Build history of the part. All positions in model axes, mm. A direction names the side the tool comes from. Coordinates: 2 decimals unless noted, no trailing zeros. Loops run counter-clockwise (first coordinate to the right, second up) from the corner with the lowest first, then second, coordinate; pieces in that order, holes last.
(1) Slice it at C-C (y = 17). Give the cut face in (x, z), and give its area (3 significant figures).
(2) Flat gauge pins, fed straight in: P1, Ø1, axis at x = 5, z = 4, coming from the -Y side; P2, Ø3, axis at x = -40.5, z = 6.5, coming from the -Y side; P3, Ø3, axis at x = -32, z = 7.5, coming from the +Y side. Where does each tip first touch, or does it go through?
(3) Slice it at B-B (z = 5). Give the number of separate pieces and of enclosed holes in the cut face, and give its area (3 significant figures).
(4) Slice it at A-A (x = 0). Give the cut face in (y, z).
(5) Slice it at D-D (x = 12.5). Give the cut face in (y, z).
(6) Two-plate mould, pull along Y, no slides. Class faces 5 (the face through (7.17, -39.42, 4.93)), 6 (the face through (30.656, -26.098, 4.93)), 7 (the face through (20, -1, 0)), 8 (the face through (12.03, 37.84, 4.93)): pulls with the +Y half, pulls with the -Y half, needs draft (parallel to the pull), parting line crosses it, or undercut.
(7) Tool access for faces 1 (the face through (22.336, -39.066, 4.93)), 2 (the face through (26.67, 29.19, 4.93)), 3 (the face through (-39, -8.5, 5)), 4 (the face through (-15, 19.8, 5.1)): list every direction of +Z, -Z, +X, -X, +Y, -Y with a clear straight run to the whole face (end or side of a thin tool).
(8) Wall check: L1, parallel to Y at x = -3.5, z = 6; L2, parallel to X at y = -23.5, z = 5.75; L3, parallel to X at y = 1, z = 7.5. Give the ranges that are in metal, low to high.
from build123d import *

# Parameters (mm, degrees)
SALIENTE_EXTRUIR3_DEPTH = 10
CROQUIS2_R              = 16
CROQUIS2_R_2            = 4
CROQUIS2_R_3            = 3.3
CORTAR_EXTRUIR1_DEPTH   = 65.926288457


with BuildPart() as part:
    # Croquis1 → Saliente-Extruir3 (new body)
    with BuildSketch(Plane.XY):
        with BuildLine():
            Line((-45, -8.5), (-32.403703492, -8.5))
            ThreePointArc((-32.403703492, -8.5), (-33.5, 0), (-32.403703492, 8.5))
            Line((-32.403703492, 8.5), (-45, 8.5))
            Line((-45, 8.5), (-45, -8.5))
        make_face()
        with BuildLine():
            ThreePointArc((-32.403703492, 8.5), (-33.5, 0), (-32.403703492, -8.5))
            Line((-32.403703492, -8.5), (-30, -8.5))
            Line((-30, -8.5), (-30, 8.5))
            Line((-30, 8.5), (-32.403703492, 8.5))
        make_face()
        with BuildLine():
            Line((3.308657049, -32.730762114), (26.691342951, -19.230762114))
            Line((26.691342951, -19.230762114), (27.021052668, -19.801836095))
            ThreePointArc((27.021052668, -19.801836095), (31.839089688, -10.417406962), (33.5, 0))
            ThreePointArc((33.5, 0), (30.916118508, 12.901302895), (23.563067678, 23.812430401))
            Line((23.563067678, 23.812430401), (22.361215932, 21.730762114))
            Line((22.361215932, 21.730762114), (7.638784068, 30.230762114))
            Line((7.638784068, 30.230762114), (8.840635814, 32.312430401))
            ThreePointArc((8.840635814, 32.312430401), (-16.75, 29.011851027), (-32.403703492, 8.5))
            Line((-32.403703492, 8.5), (-30, 8.5))
            Line((-30, 8.5), (-30, -8.5))
            Line((-30, -8.5), (-32.403703492, -8.5))
            ThreePointArc((-32.403703492, -8.5), (-18.9906271, -27.597211496), (3.638366766, -33.301836095))
            Line((3.638366766, -33.301836095), (3.308657049, -32.730762114))
        make_face()
        with BuildLine():
            Line((22.361215932, 21.730762114), (23.563067678, 23.812430401))
            ThreePointArc((23.563067678, 23.812430401), (16.75, 29.011851027), (8.840635814, 32.312430401))
            Line((8.840635814, 32.312430401), (7.638784068, 30.230762114))
            Line((7.638784068, 30.230762114), (22.361215932, 21.730762114))
        make_face()
        with BuildLine():
            ThreePointArc((8.840635814, 32.312430401), (16.75, 29.011851027), (23.563067678, 23.812430401))
            Line((23.563067678, 23.812430401), (29.861215932, 34.72114317))
            Line((29.861215932, 34.72114317), (15.138784068, 43.22114317))
            Line((15.138784068, 43.22114317), (8.840635814, 32.312430401))
        make_face()
        with BuildLine():
            Line((27.021052668, -19.801836095), (26.691342951, -19.230762114))
            Line((26.691342951, -19.230762114), (3.308657049, -32.730762114))
            Line((3.308657049, -32.730762114), (3.638366766, -33.301836095))
            ThreePointArc((3.638366766, -33.301836095), (16.75, -29.011851027), (27.021052668, -19.801836095))
        make_face()
        with BuildLine():
            Line((34.191342951, -32.22114317), (27.021052668, -19.801836095))
            ThreePointArc((27.021052668, -19.801836095), (16.75, -29.011851027), (3.638366766, -33.301836095))
            Line((3.638366766, -33.301836095), (10.808657049, -45.72114317))
            Line((10.808657049, -45.72114317), (34.191342951, -32.22114317))
        make_face()
    extrude(amount=SALIENTE_EXTRUIR3_DEPTH)

    # Croquis2 → Cortar-Extruir1 (cut, through all)
    with BuildSketch(Plane.XY.offset(10)):
        Circle(CROQUIS2_R)
        with Locations((12.5, -21.650635095)):
            Circle(CROQUIS2_R_2)
        with Locations((24.148145657, -6.470476128)):
            Circle(CROQUIS2_R_3)
        with Locations((-6.470476128, -24.148145657)):
            Circle(CROQUIS2_R_3)
        with Locations((6.470476128, 24.148145657)):
            Circle(CROQUIS2_R_3)
        with Locations((-24.148145657, 6.470476128)):
            Circle(CROQUIS2_R_3)
        with Locations((24.947836968, -29.091113341)):
            Circle(CROQUIS2_R_3)
        with Locations((12.719724694, -36.151017254)):
            Circle(CROQUIS2_R_3)
        Polygon((-19.486906027, 27.568394577), (-10.486906027, 11.979937309), (-5.213138932, 15.024748161), (-14.213138932, 30.613205429), align=None)
        with Locations((-38.701851746, 0)):
            Circle(CROQUIS2_R_3)
        with Locations((19.350925873, 33.516786786)):
            Circle(CROQUIS2_R_3)
    extrude(amount=-CORTAR_EXTRUIR1_DEPTH, mode=Mode.SUBTRACT)


solid = part.part
Response values:
1. outline: (-28.87, 0) - (-13.39, 0) - (-13.39, 10) - (-28.87, 10) - close; (-6.35, 0) - (28.87, 0) - (28.87, 10) - (-6.35, 10) - close
1. area: 507 mm2
2. P1: stops at y = -36.53
2. P2: stops at y = -8.5
2. P3: stops at y = 13.86
3. separate pieces: 1
3. enclosed holes: 9
3. area: 3,030 mm2
4. outline: (-33.5, 0) - (-16, 0) - (-16, 10) - (-33.5, 10) - close; (16, 0) - (33.5, 0) - (33.5, 10) - (16, 10) - close
5. outline: (-44.74, 0) - (-39.44, 0) - (-39.44, 10) - (-44.74, 10) - close; (-32.86, 0) - (-25.65, 0) - (-25.65, 10) - (-32.86, 10) - close; (-17.65, 0) - (-9.99, 0) - (-9.99, 10) - (-17.65, 10) - close; (9.99, 0) - (38.65, 0) - (38.65, 10) - (9.99, 10) - close
6. face 5: pulls with the -Y half
6. face 6: undercut
6. face 7: needs draft
6. face 8: pulls with the +Y half
7. face 1: +Z, -Z, +X, -Y
7. face 2: +Z, -Z, +X
7. face 3: +Z, -Z, -X, -Y
7. face 4: +Z, -Z
8. L1: y = -33.32 to -25.59, -22.71 to -15.61, 15.61 to 33.32
8. L2: x = -23.87 to -9.71, -3.23 to 8.95, 16.05 to 29.16
8. L3: x = -45 to -41.85, -35.56 to -15.97, 15.97 to 33.49
